from build123d import *

# Parameters (mm, degrees)
SKETCH1_W                    = 105
SKETCH1_H                    = 905.2
BASE_FLANGE1_DEPTH           = 1
EDGE_FLANGE1_STRIP_W         = 6
EDGE_FLANGE1_STRIP_H         = 1
EDGE_FLANGE1_STRIP_CUT_DEPTH = 905.2
EDGE_FLANGE1_DEPTH           = 905.2
EDGE_FLANGE2_STRIP_W         = 6
EDGE_FLANGE2_STRIP_H         = 1
EDGE_FLANGE2_STRIP_CUT_DEPTH = 905.2
EDGE_FLANGE2_DEPTH           = 905.2
SKETCH19_R                   = 2.5
CUT_EXTRUDE2_DEPTH           = 10
CUT_EXTRUDE3_START           = -905.2
CUT_EXTRUDE3_DEPTH           = 20.5


# Read off the part's stored shape, not the designer's step: Cut-Extrude3
# Sheet-metal steps are written as plain solids
with BuildPart() as part:
    # Sketch1 → Base-Flange1 (new body)
    with BuildSketch(Plane(origin=(0, 0, 0), x_dir=(1, 0, 0), z_dir=(0, 1, 0))):
        with Locations((52.5, 452.6)):
            Rectangle(SKETCH1_W, SKETCH1_H)
    extrude(amount=-BASE_FLANGE1_DEPTH)

    # Edge-Flange1 strip (across the edge) → Edge-Flange1 strip cut (cut)
    with BuildSketch(Plane(origin=(105, 0, 0), x_dir=(-1, 0, 0), z_dir=(0, 0, -1))):
        with Locations((-1, -0.5)):
            Rectangle(EDGE_FLANGE1_STRIP_W, EDGE_FLANGE1_STRIP_H)
    extrude(amount=EDGE_FLANGE1_STRIP_CUT_DEPTH, mode=Mode.SUBTRACT)

    # Edge-Flange1 section (across the edge) → Edge-Flange1 (add)
    with BuildSketch(Plane(origin=(105, 0, 0), x_dir=(-1, 0, 0), z_dir=(0, 0, -1))):
        with BuildLine():
            Line((0, 1), (0, 19))
            Line((0, 19), (1, 19))
            Line((1, 19), (1, 1))
            ThreePointArc((1, 1), (1.292893219, 0.292893219), (2, 0))
            Line((2, 0), (2, -1))
            ThreePointArc((2, -1), (0.585786438, -0.414213562), (0, 1))
        make_face()
    extrude(amount=EDGE_FLANGE1_DEPTH)

    # Edge-Flange2 strip (across the edge) → Edge-Flange2 strip cut (cut)
    with BuildSketch(Plane(origin=(104, 19, 0), x_dir=(0, -1, 0), z_dir=(0, 0, -1))):
        with Locations((-1, -0.5)):
            Rectangle(EDGE_FLANGE2_STRIP_W, EDGE_FLANGE2_STRIP_H)
    extrude(amount=EDGE_FLANGE2_STRIP_CUT_DEPTH, mode=Mode.SUBTRACT)

    # Edge-Flange2 section (across the edge) → Edge-Flange2 (add)
    with BuildSketch(Plane(origin=(104, 19, 0), x_dir=(0, -1, 0), z_dir=(0, 0, -1))):
        with BuildLine():
            Line((0, 1), (0, 12))
            Line((0, 12), (1, 12))
            Line((1, 12), (1, 1))
            ThreePointArc((1, 1), (1.292893219, 0.292893219), (2, 0))
            Line((2, 0), (2, -1))
            ThreePointArc((2, -1), (0.585786438, -0.414213562), (0, 1))
        make_face()
    extrude(amount=EDGE_FLANGE2_DEPTH)

    # Sketch19 → Cut-Extrude2 (cut)
    with BuildSketch(Plane(origin=(0, 19, 0), x_dir=(1, 0, 0), z_dir=(0, 1, 0))):
        with Locations(Location((98, 63, 0), (0, 0, 180))):
            Circle(SKETCH19_R)
        with Locations(Location((98, 108, 0), (0, 0, 180))):
            Circle(SKETCH19_R)
        with Locations(Location((98, 276, 0), (0, 0, 180))):
            Circle(SKETCH19_R)
        with Locations(Location((98, 444, 0), (0, 0, 180))):
            Circle(SKETCH19_R)
        with Locations(Location((98, 612, 0), (0, 0, 180))):
            Circle(SKETCH19_R)
        with Locations(Location((98, 780, 0), (0, 0, 180))):
            Circle(SKETCH19_R)
    extrude(amount=-CUT_EXTRUDE2_DEPTH, mode=Mode.SUBTRACT)

    # Cut-Extrude3 outline → Cut-Extrude3 (cut)
    with BuildSketch(Plane.XY.offset(CUT_EXTRUDE3_START)):
        with BuildLine():
            ThreePointArc((104, 1), (103.707106781, 0.292893219), (103, 0))
            Line((103, 0), (103, -1))
            ThreePointArc((103, -1), (104.414213562, -0.414213562), (105, 1))
            Line((105, 1), (105, 17))
            ThreePointArc((105, 17), (104.414213562, 18.414213562), (103, 19))
            Line((103, 19), (92, 19))
            Line((92, 19), (92, 18))
            Line((92, 18), (103, 18))
            ThreePointArc((103, 18), (103.707106781, 17.707106781), (104, 17))
            Line((104, 17), (104, 1))
        make_face()
    extrude(amount=CUT_EXTRUDE3_DEPTH, mode=Mode.SUBTRACT)


solid = part.part
Verification items for the finished model (mm, model axes). Round coordinates to 2 decimals unless told otherwise and drop trailing zeros. Loops run counter-clockwise (first coordinate to the right, second up) from the corner with the lowest first, then second, coordinate; pieces in that order, holes last. Notation, with made-up numbers: (-17.75, -15.5) - (-8.75, -15.5) arc R18 ccw to (-8.75, 2.5) - close; hole circle Ø7 at (11.5, -33). An arc over 180 degrees is marked (long way). Answer in a Markdown table with one row per item. Add a question column.
Q1. Section check C-C on x = 61.5. Enter the section's corners in (y, z).
Q2. Release check for a two-part mould opening along Y. For faces 1 (the face through (104, 9, -436)), 2 (the face through (105, 9, -436)), 3 (the face through (51, -1, -459)) record: pulls with the +Y half, pulls with the -Y half, needs draft (parallel to the pull), parting line crosses it, or undercut.
Q3. Section check A-A on z = -149. Enter the section's corners in (x, y), plus the area to 3 significant figures.
Q4. Section check B-B on y = 13.5. Enter the section's corners in (x, z).
Q5. Material ranges on line 1 (X direction, y = 18.7, z = -612); line 2 (Y direction, x = 73, z = -384); line 3 (X direction, y = 12.5, z = -748.5), recorded low to high.
Q6. Gauge pin test, flat ends, axial feed: pin 1 (3 mm diameter, centred on y = 5, z = -255.5, fed in from -X); pin 2 (4 mm diameter, centred on x = 98, z = -444, fed in from +Y); pin 3 (12 mm diameter, centred on x = 11, y = 9, fed in from -Z); pin 4 (0.8 mm diameter, centred on y = 18.5, z = -349, fed in from -X). Record the tip position at first contact, or that the pin passes through.
Found:
| question | item | result |
|---|---|---|
| 1 | outline | (-1, -905.2) - (0, -905.2) - (0, 0) - (-1, 0) - close |
| 2 | face 1 | undercut |
| 2 | face 2 | needs draft |
| 2 | face 3 | pulls with the -Y half |
| 3 | outline | (0, -1) - (103, -1) arc R2 ccw to (105, 1) - (105, 17) arc R2 ccw to (103, 19) - (92, 19) - (92, 18) - (103, 18) arc R1 cw to (104, 17) - (104, 1) arc R1 cw to (103, 0) - (0, 0) - close |
| 3 | area | 135 mm² |
| 4 | outline | (104, -884.7) - (105, -884.7) - (105, 0) - (104, 0) - close |
| 5 | line 1 | x = 92 to 95.5, 100.5 to 104.05 |
| 5 | line 2 | y = -1 to 0 |
| 5 | line 3 | x = 104 to 105 |
| 6 | pin 1 | stops at x = 104 |
| 6 | pin 2 | stops at y = 0 |
| 6 | pin 3 | passes through |
| 6 | pin 4 | stops at x = 92 |
